Check sheet for the modelled part. Datum: model origin and axes. Units: mm. Face numbers are marked on the shaded views. A direction names the side the tool comes from. Round coordinates to 2 decimals unless told otherwise and drop trailing zeros. Order: outer loops, then holes, each group sorted by start corner. A loop starts at its lowest first (then second) coordinate and runs counter-clockwise, first axis right, second up. Notation, with made-up numbers: (15.25, -19) -> (66.25, -19) arc R29 ccw to (66.25, 1) -> close; hole circle Ø1 at (23, 46.25). An arc over 180 degrees is marked (long way). Answer in a Markdown table with one row per item.
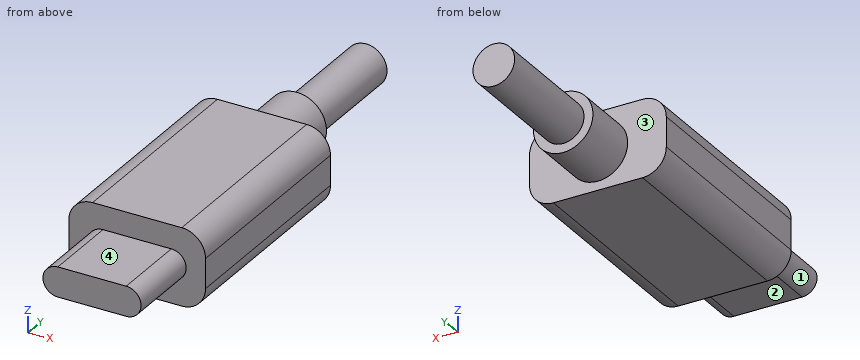
from build123d import *

# Parameters (mm, degrees)
PAD_DEPTH    = 6.5
SKETCH001_W  = 11.5
SKETCH001_H  = 6.5
PAD001_DEPTH = 18
FILLET_R     = 2
SKETCH002_R  = 2.5
PAD002_DEPTH = 5
SKETCH003_R  = 1.75
PAD003_DEPTH = 10


with BuildPart() as part:
    # Sketch → Pad (new body)
    with BuildSketch(Plane.XZ):
        with BuildLine():
            ThreePointArc((-2.875, 1.25), (-4.125, 0), (-2.875, -1.25))
            Line((-2.875, -1.25), (2.875, -1.25))
            ThreePointArc((2.875, -1.25), (4.125, 0), (2.875, 1.25))
            Line((2.875, 1.25), (-2.875, 1.25))
        make_face()
    extrude(amount=PAD_DEPTH)

    # Sketch001 → Pad001 (join)
    with BuildSketch(Plane.XZ):
        Rectangle(SKETCH001_W, SKETCH001_H)
    extrude(amount=-PAD001_DEPTH)

    # Fillet
    fillet_edges = [part.edges().sort_by_distance(p)[0] for p in [
        (-5.75, 9, 3.25),
        (5.75, 9, 3.25),
        (5.75, 9, -3.25),
        (-5.75, 9, -3.25),
    ]]
    fillet(fillet_edges, radius=FILLET_R)

    # Sketch002 (on Face5 of Fillet) → Pad002 (join)
    with BuildSketch(Plane(origin=(0, 18, 0), x_dir=(1, 0, 0), z_dir=(0, 1, 0))):
        Circle(SKETCH002_R)
    extrude(amount=PAD002_DEPTH)

    # Sketch003 (on Face17 of Pad002) → Pad003 (join)
    with BuildSketch(Plane(origin=(0, 23, 0), x_dir=(1, 0, 0), z_dir=(0, 1, 0))):
        Circle(SKETCH003_R)
    extrude(amount=PAD003_DEPTH)


solid = part.part
Item 1: Cross-section at C-C (x = 0). Record the boundary of the cut face in (y, z), and give its area (3 significant figures).
Result sheet:
| item | result |
|---|---|
| outline | (-6.5, -1.25) -> (0, -1.25) -> (0, -3.25) -> (18, -3.25) -> (18, -2.5) -> (23, -2.5) -> (23, -1.75) -> (33, -1.75) -> (33, 1.75) -> (23, 1.75) -> (23, 2.5) -> (18, 2.5) -> (18, 3.25) -> (0, 3.25) -> (0, 1.25) -> (-6.5, 1.25) -> close |
| area | 193 mm^2 |
Item 2: Scan lines: line 1 (Y direction, x = -1, z = 1.75); line 2 (Y direction, x = 2.5, z = 1.5); line 3 (Z direction, x = 0, y = 20.5). Record each from-to range of solid material in increasing order. Write a range as [from, to].
Result sheet:
| item | result |
|---|---|
| line 1 | y = [0, 23] |
| line 2 | y = [0, 18] |
| line 3 | z = [-2.5, 2.5] |
Item 3: Cross-section at B-B (y = 11). Record the boundary of the cut face in (x, z), and give its area (3 significant figures).
Result sheet:
| item | result |
|---|---|
| outline | (-5.75, -1.25) arc R2 ccw to (-3.75, -3.25) -> (3.75, -3.25) arc R2 ccw to (5.75, -1.25) -> (5.75, 1.25) arc R2 ccw to (3.75, 3.25) -> (-3.75, 3.25) arc R2 ccw to (-5.75, 1.25) -> close |
| area | 71.3 mm^2 |
Item 4: Cross-section at A-A (z = 0). Record the boundary of the cut face in (x, y) (3 decimals), and give its area (3 significant figures).
Result sheet:
| item | result |
|---|---|
| outline | (-5.75, 0) -> (-4.125, 0) -> (-4.125, -6.5) -> (4.125, -6.5) -> (4.125, 0) -> (5.75, 0) -> (5.75, 18) -> (2.5, 18) -> (2.5, 23) -> (1.75, 23) -> (1.75, 33) -> (-1.75, 33) -> (-1.75, 23) -> (-2.5, 23) -> (-2.5, 18) -> (-5.75, 18) -> close |
| area | 321 mm^2 |
Item 5: Cross-section at D-D (y = 29). Record the boundary of the cut face in (x, z).
Result sheet:
| item | result |
|---|---|
| outline | circle Ø3.5 at (0, 0) |
Item 6: Set-up check for the marked faces 1, 2, 3 and 4: record each of +Z, -Z, +X, -X, +Y, -Y from which the full face is reachable in a straight line by a thin tool's end or side.
Result sheet:
| item | result |
|---|---|
| face 1 | -X, -Y |
| face 2 | -Z, +X, -X, -Y |
| face 3 | +Y |
| face 4 | +Z, +X, -X, -Y |
Item 7: Depth check by flat-ended pin: P1, Ø3, axis at x = 2, y = 24, coming from the -Z side; P2, Ø3, axis at x = 0, y = -4.5, coming from the +Z side; P3, Ø5, axis at x = 0, y = 26.5, coming from the +Z side. Enter the tip coordinate at first touch or a pass-through.
Result sheet:
| item | result |
|---|---|
| P1 | stops at z = -2.34 |
| P2 | stops at z = 1.25 |
| P3 | stops at z = 1.75 |
